For this review, use the dimensioned drawing (mm, ordinates from the lowest corner) and the shaded views. Coordinates: 2 decimals unless noted, no trailing zeros. Loops run counter-clockwise (first coordinate to the right, second up) from the corner with the lowest first, then second, coordinate; pieces in that order, holes last. Notation, with made-up numbers: M 38,-30.75 L 67,-30.75 A26 cw 67,-6.75 Z; hole C 72.25,46.25 d6. An arc over 180 degrees is marked long. Write item = value, one per line. Start each with the question number.
Q1. We need section A-A on z = 1.5. Give the boundary of the cut face in (x, y).
Q2. We need section B-B on y = 19. Give the boundary of the cut face in (x, z), and give its area (3 significant figures).
Q3. We need section C-C on x = 17.5. Give the boundary of the cut face in (y, z).
Q4. Clearance check with a flat-ended pin moving along its axis: pin 1 Ø1.5 at (x, z) = (9, 2) entering from -Y. State where the tip first meets the part, or that it passes through.
Q5. Mouldability with a two-part tool opening along Z and no side actions: class the marked faces 1 and 2 as released by +Z, released by -Z, zero draft, split by the parting line, or undercut.
Q6. Wall thickness on probe 1 along X at (y, z) = (6, 0.7); probe 2 along X at (y, z) = (5.5, 0.25); probe 3 along Y at (x, z) = (13.5, 1): over which ranges is each line inside the solid? List them lowest first.
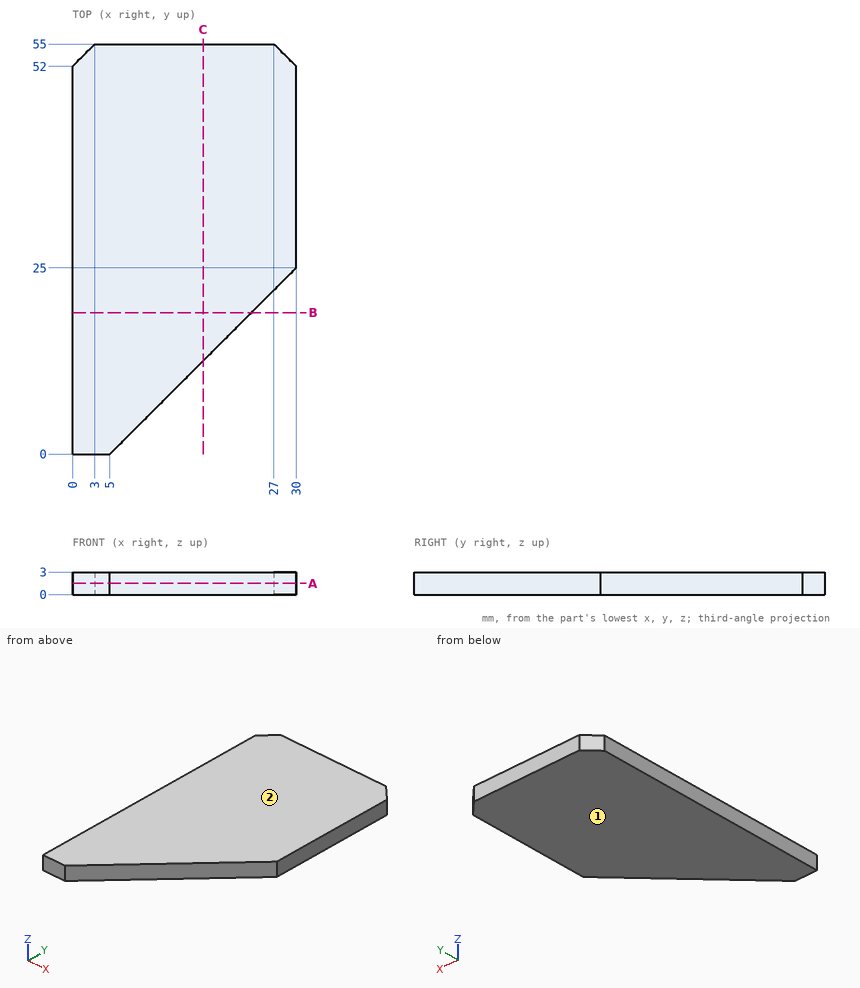
Returned:
q1.outline = M 0,0 L 5,0 L 30,25 L 30,52 L 27,55 L 3,55 L 0,52 Z
q2.outline = M 0,0 L 24,0 L 24,3 L 0,3 Z
q2.area = 72.0 mm^2
q3.outline = M 12.5,0 L 55,0 L 55,3 L 12.5,3 Z
q4.pin_1 = 3.25
q5.face_1 = released by -Z
q5.face_2 = released by +Z
q6.probe_1 = 0 to 11
q6.probe_2 = 0 to 10.5
q6.probe_3 = 8.5 to 55
